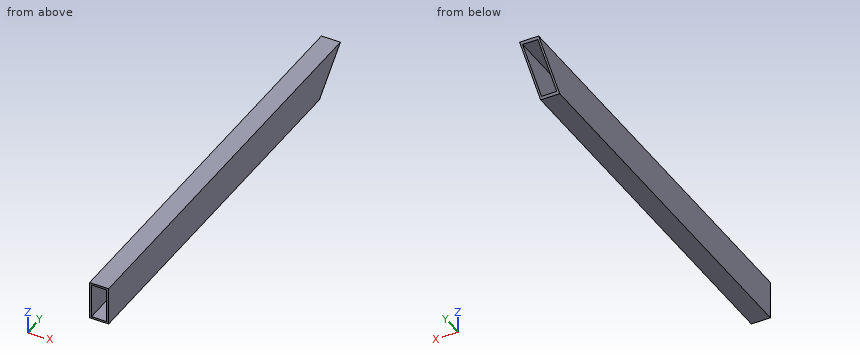
Autodesk Inventor part; units mm, degrees
ref_plane "YZ Plane" through (0, 0, 0) normal (1, 0, 0) x (0, 1, 0)
ref_plane "XZ Plane" through (0, 0, 0) normal (0, 1, 0) x (-1, 0, 0)
ref_plane "XY Plane" through (0, 0, 0) normal (0, 0, 1) x (1, 0, 0)
sketch "Sketch1" plane through (0, 0, 0) normal (0, 1, 0) x (-1, 0, 0)
  line L0 (-9.4777, 15.0257) -> (40.5223, 15.0257)
  line L1 (40.5223, 15.0257) -> (40.5223, -84.9743)
  line L2 (40.5223, -84.9743) -> (-9.4777, -84.9743)
  line L3 (-9.4777, -84.9743) -> (-9.4777, 15.0257)
  line L4 (35.5223, 10.0257) -> (-4.4777, 10.0257)
  line L5 (-4.4777, 10.0257) -> (-4.4777, -79.9743)
  line L6 (-4.4777, -79.9743) -> (35.5223, -79.9743)
  line L7 (35.5223, -79.9743) -> (35.5223, 10.0257)
  point P0 (0, 0)
  point P1 (0, 0)
  dimension "d0" = 50
  dimension "d1" = 100
  dimension "d2" = 5
  dimension "d3" = 90
  dimension "d4" = 5
  dimension "d5" = 40
extrude "Extrusion1" add sketch "Sketch1" along normal blind 1100
sketch "Sketch2" plane through (9.4777, 0, 15.0257) normal (1, 0, 0) x (0, 0, -1)
  line L0 (-0.8068, 1100.2585) -> (100, 999.4516)
  line L1 (100, 0) -> (100, 1100)
  line L2 (-0.8068, 1100.2585) -> (141.7556, 1100.2585) construction
  line L3 (100, 999.4516) -> (100, 1100)
  line L4 (0, 0) -> (0, 1100)
  line L5 (100, 1100) -> (0, 1100)
  point P0 (15.0257, 0)
  point P1 (0, 1099.4516)
  dimension "d8" = 45
extrude "Extrusion2" cut sketch "Sketch2" against normal blind 1100
properties part number "PerfilV2"
Geometry: final body of the model. Coordinates: model frame, mm. Coordinates: 2 decimals unless noted, no trailing zeros. Order: outer loops, then holes, each group sorted by start corner. A loop starts at its lowest first (then second) coordinate and runs counter-clockwise, first axis right, second up.
(1) First-contact query: pin 1 (6 mm diameter, centred on x = -30, z = -38.5, fed in from -Y). Flat tip, straight axial feed; report the tip coordinate or a pass-through.
(2) Section query B-B (x = -6.5). Return the cut outline in (y, z), plus the area to 3 significant figures.
(3) Section query C-C (y = 266.5). Return the cut outline in (x, z), plus the area to 3 significant figures.
(4) Section query A-A (z = -32). Return the cut outline in (x, y).
(5) Material intervals for probe 1 along Z at (x, y) = (-20.5, 264.5); probe 2 along X at (y, z) = (565.5, -17); probe 3 along Y at (x, z) = (-36, -30), sorted ascending.
Solution:
1. pin 1: passes through
2. outline: (0, -84.97) - (999.45, -84.97) - (1004.45, -79.97) - (0, -79.97) - close; (0, 10.03) - (1094.45, 10.03) - (1099.45, 15.03) - (0, 15.03) - close
2. area: 10,500 mm2
3. outline: (-40.52, -84.97) - (9.48, -84.97) - (9.48, 15.03) - (-40.52, 15.03) - close; hole (-35.52, -79.97) - (4.48, -79.97) - (4.48, 10.03) - (-35.52, 10.03) - close
3. area: 1,400 mm2
4. outline: (-40.52, 0) - (-35.52, 0) - (-35.52, 1052.43) - (-40.52, 1052.43) - close; (4.48, 0) - (9.48, 0) - (9.48, 1052.43) - (4.48, 1052.43) - close
5. probe 1: z = -84.97 to -79.97, 10.03 to 15.03
5. probe 2: x = -40.52 to -35.52, 4.48 to 9.48
5. probe 3: y = 0 to 1054.43
